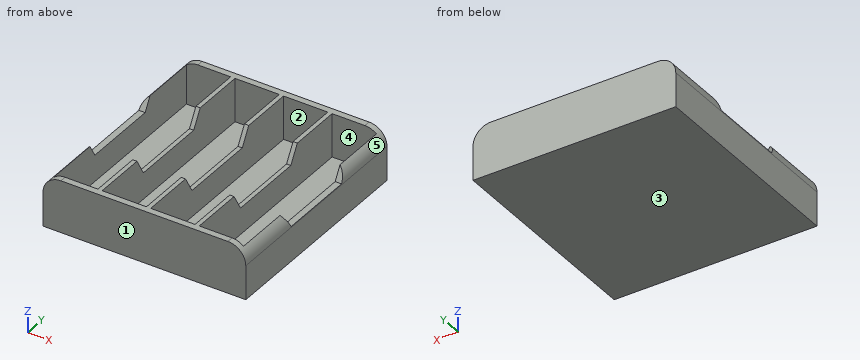
```python
from build123d import *

# Parameters (mm, degrees)
SKETCH1_W               = 47.52
SKETCH1_H               = 50.5
BOSS_EXTRUDE1_DEPTH     = 2
BOSS_EXTRUDE2_DEPTH     = 50.5
SKETCH3_W               = 10.38
SKETCH3_H               = 47.5
CUT_EXTRUDE1_DEPTH      = 10.2
CUT_EXTRUDE2_DEPTH      = 37.755137056
CUT_EXTRUDE2_DEPTH_BACK = 37.755137056


with BuildPart() as part:
    # Sketch1 → Boss-Extrude1 (new body)
    with BuildSketch(Plane.XY):
        Rectangle(SKETCH1_W, SKETCH1_H)
    extrude(amount=BOSS_EXTRUDE1_DEPTH)

    # Sketch2 → Boss-Extrude2 (add)
    with BuildSketch(Plane.XZ.offset(25.25)):
        with BuildLine():
            Line((-19.56, 12.2), (19.56, 12.2))
            ThreePointArc((19.56, 12.2), (22.529848481, 10.969848481), (23.76, 8))
            Line((23.76, 8), (23.76, 2))
            Line((23.76, 2), (-23.76, 2))
            Line((-23.76, 2), (-23.76, 8))
            ThreePointArc((-23.76, 8), (-22.529848481, 10.969848481), (-19.56, 12.2))
        make_face()
    extrude(amount=-BOSS_EXTRUDE2_DEPTH)

    # Sketch3 → Cut-Extrude1 (cut)
    with BuildSketch(Plane.XY.offset(12.2)):
        with Locations((-17.07, 0)):
            Rectangle(SKETCH3_W, SKETCH3_H)
        with Locations((-5.69, 0)):
            Rectangle(SKETCH3_W, SKETCH3_H)
        with Locations((5.69, 0)):
            Rectangle(SKETCH3_W, SKETCH3_H)
        with Locations((17.07, 0)):
            Rectangle(SKETCH3_W, SKETCH3_H)
    extrude(amount=-CUT_EXTRUDE1_DEPTH, mode=Mode.SUBTRACT)

    # Sketch4 → Cut-Extrude2 (cut, two sides: drawn at the far end of the back side and taken through both)
    with BuildSketch(Plane(origin=(0, 0, 0), x_dir=(0, 0, -1), z_dir=(1, 0, 0)).offset(-CUT_EXTRUDE2_DEPTH_BACK)):
        Polygon((-17.2, -14.196152423), (-17.2, 14.196152423), (-8.2, 9), (-8.2, -9), align=None)
    extrude(amount=CUT_EXTRUDE2_DEPTH + CUT_EXTRUDE2_DEPTH_BACK, mode=Mode.SUBTRACT)


solid = part.part
```
Geometry: final body of the model. Coordinates: model frame, mm. Face numbers are marked on the shaded views. A direction names the side the tool comes from. Round coordinates to 2 decimals unless told otherwise and drop trailing zeros. Order: outer loops, then holes, each group sorted by start corner. A loop starts at its lowest first (then second) coordinate and runs counter-clockwise, first axis right, second up. Notation, with made-up numbers: (88.5, 27) -> (140.5, 27) arc R15 cw to (140.5, 37) -> close; hole circle Ø10 at (28, 59). An arc over 180 degrees is marked (long way). Use CSV: the item, a comma, the result in double quotes. Start each with the question number.
1) Section C-C (x = -1.5). Return the cut outline in (y, z), and give its area (3 significant figures).
2) Material intervals for line 1 along X through (y, z) = (14, 3.25); line 2 along Y through (x, z) = (-20, 3.5); line 3 along Z through (x, y) = (15, 17), sorted ascending. Write a range as from..to.
3) Section A-A (z = 7). Return the cut outline in (x, y), and give its area (3 significant figures).
4) First-contact query: pin 1 Ø1.1 at (x, y) = (11.5, 3) entering from +Z; pin 2 Ø3 at (x, y) = (-4.5, 6) entering from +Z. Flat tips, straight axial feed; report the tip coordinate or a pass-through.
5) Set-up query: the marked faces 4 and 5. Return all of +Z, -Z, +X, -X, +Y, -Y with unobstructed straight access to the full face (end or side cutting, diameter ignored); none if empty.
6) Section B-B (y = -16.5). Return the cut outline in (x, z), and give its area (3 significant figures).
7) Draft query along Y for the marked faces 1, 2 and 3. Return one class per face: +Y half, -Y half, draft (parallel to the pull), parting line (faces both ways), or undercut.
8) Section D-D (y = -7.5). Return the cut outline in (x, z).
Returned:
1,outline,"(-25.25, 0) -> (25.25, 0) -> (25.25, 12.2) -> (23.75, 12.2) -> (23.75, 2) -> (-23.75, 2) -> (-23.75, 12.2) -> (-25.25, 12.2) -> close"
1,area,"132 mm²"
2,line 1,"x = -23.76..-22.26, -11.88..-10.88, -0.5..0.5, 10.88..11.88, 22.26..23.76"
2,line 2,"y = -25.25..-23.75, 23.75..25.25"
2,line 3,"z = 0..2"
3,outline,"(-23.76, -25.25) -> (23.76, -25.25) -> (23.76, 25.25) -> (-23.76, 25.25) -> close; hole (-22.26, -23.75) -> (-11.88, -23.75) -> (-11.88, 23.75) -> (-22.26, 23.75) -> close; hole (-10.88, -23.75) -> (-0.5, -23.75) -> (-0.5, 23.75) -> (-10.88, 23.75) -> close; hole (0.5, -23.75) -> (10.88, -23.75) -> (10.88, 23.75) -> (0.5, 23.75) -> close; hole (11.88, -23.75) -> (22.26, -23.75) -> (22.26, 23.75) -> (11.88, 23.75) -> close"
3,area,"428 mm²"
4,pin 1,"stops at z = 8.2"
4,pin 2,"stops at z = 2"
5,face 4,"+Z"
5,face 5,"+Z, +X, +Y, -Y"
6,outline,"(-23.76, 0) -> (23.76, 0) -> (23.76, 8) arc R4.2 ccw to (22.26, 11.22) -> (22.26, 2) -> (11.88, 2) -> (11.88, 12.2) -> (10.88, 12.2) -> (10.88, 2) -> (0.5, 2) -> (0.5, 12.2) -> (-0.5, 12.2) -> (-0.5, 2) -> (-10.88, 2) -> (-10.88, 12.2) -> (-11.88, 12.2) -> (-11.88, 2) -> (-22.26, 2) -> (-22.26, 11.22) arc R4.2 ccw to (-23.76, 8) -> close"
6,area,"150 mm²"
7,face 1,"-Y half"
7,face 2,"undercut"
7,face 3,"draft"
8,outline,"(-23.76, 0) -> (23.76, 0) -> (23.76, 8) arc R4.2 ccw to (23.76, 8.2) -> (22.26, 8.2) -> (22.26, 2) -> (11.88, 2) -> (11.88, 8.2) -> (10.88, 8.2) -> (10.88, 2) -> (0.5, 2) -> (0.5, 8.2) -> (-0.5, 8.2) -> (-0.5, 2) -> (-10.88, 2) -> (-10.88, 8.2) -> (-11.88, 8.2) -> (-11.88, 2) -> (-22.26, 2) -> (-22.26, 8.2) -> (-23.76, 8.2) arc R4.2 ccw to (-23.76, 8) -> close"
